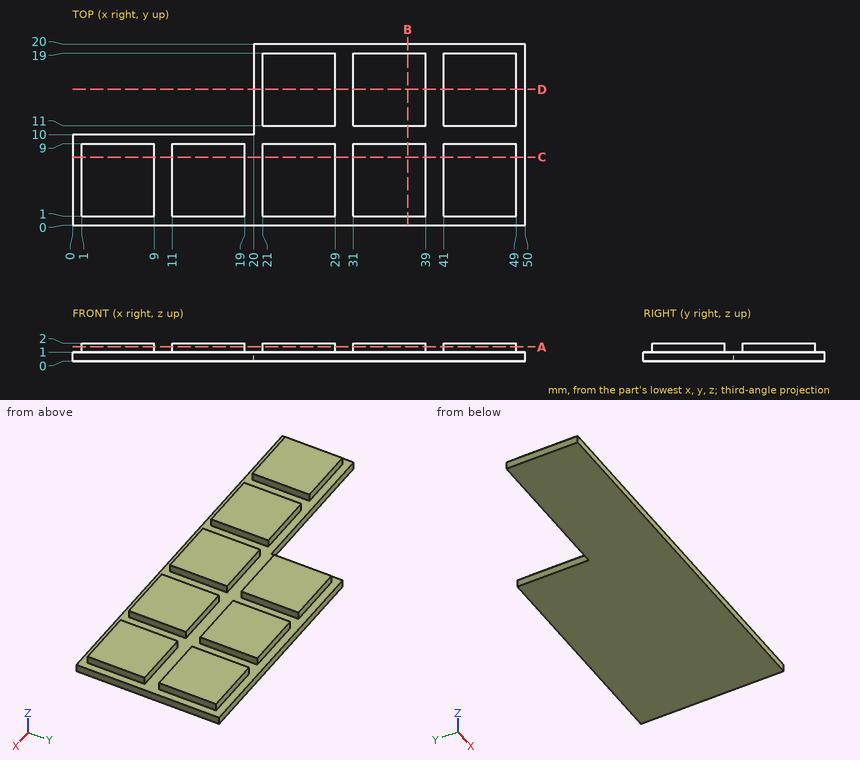
Drawing for the job (mm, zero at the part's lowest x, y, z). Round coordinates to 2 decimals unless told otherwise and drop trailing zeros. Loops run counter-clockwise (first coordinate to the right, second up) from the corner with the lowest first, then second, coordinate; pieces in that order, holes last. Notation, with made-up numbers: (9.25, 81.5) - (39.25, 81.5) arc R19 ccw to (39.25, 114.5) - close; hole circle Ø10 at (3.5, 80). An arc over 180 degrees is marked (long way). Return JSON: item names as keys, results as strings. Group by question number.
Q1. Band-saw the part on D-D on y = 15. Give the cut face in (x, z).
Q2. Drill centre lines: line 1 along X through (y, z) = (11.75, 1.85); line 2 along X through (y, z) = (7.5, 1.6); line 3 along Y through (x, z) = (35, 1.75). Where is each one in solid material? Low to high. Write a range as [from, to].
Q3. Band-saw the part on C-C on y = 7.5. Give the cut face in (x, z), plus the area to 3 significant figures.
Q4. Flat gauge pins, fed straight in: pin 1 Ø1.1 at (x, z) = (16.5, 1.5) entering from +Y; pin 2 Ø0.8 at (x, z) = (36, 1.5) entering from -Y; pin 3 Ø0.8 at (y, z) = (3.5, 1.5) entering from -X. Where does each tip first touch, or does it go through?
Q5. Band-saw the part on A-A on z = 1.6. Give the number of separate pieces and of enclosed holes in the cut face, plus the area to 3 significant figures.
Q6. Band-saw the part on B-B on x = 37. Give the cut face in (y, z), plus the area to 3 significant figures.
Solutions:
{
 "1": {"outline": "(20, 0) - (50, 0) - (50, 1) - (49, 1) - (49, 2) - (41, 2) - (41, 1) - (39, 1) - (39, 2) - (31, 2) - (31, 1) - (29, 1) - (29, 2) - (21, 2) - (21, 1) - (20, 1) - close"},
 "2": {"line 1": "x = [21, 29], [31, 39], [41, 49]", "line 2": "x = [1, 9], [11, 19], [21, 29], [31, 39], [41, 49]", "line 3": "y = [1, 9], [11, 19]"},
 "3": {"outline": "(0, 0) - (50, 0) - (50, 1) - (49, 1) - (49, 2) - (41, 2) - (41, 1) - (39, 1) - (39, 2) - (31, 2) - (31, 1) - (29, 1) - (29, 2) - (21, 2) - (21, 1) - (19, 1) - (19, 2) - (11, 2) - (11, 1) - (9, 1) - (9, 2) - (1, 2) - (1, 1) - (0, 1) - close", "area": "90.0 mm^2"},
 "4": {"pin 1": "stops at y = 10", "pin 2": "stops at y = 1", "pin 3": "stops at x = 1"},
 "5": {"separate pieces": "8", "enclosed holes": "0", "area": "512 mm^2"},
 "6": {"outline": "(0, 0) - (20, 0) - (20, 1) - (19, 1) - (19, 2) - (11, 2) - (11, 1) - (9, 1) - (9, 2) - (1, 2) - (1, 1) - (0, 1) - close", "area": "36.0 mm^2"}
}
